CAD build for the part. Positions are in the model's coordinates, mm. Face numbers are marked on the shaded views. Give positions to 0.01 mm unless a question says otherwise; leave off trailing zeros. Answer as CSV lines item,"result".
from build123d import *

# Parameters (mm, degrees)
SKETCH_R        = 22.6
SKETCH_R_2      = 14
SKETCH_R_3      = 2.5
PAD_DEPTH       = 13
SKETCH001_R     = 27.5
SKETCH001_R_2   = 22.5
PAD001_DEPTH    = 2
CHAMFER_SIZE    = 0.5
CHAMFER001_SIZE = 1
CHAMFER002_SIZE = 0.5
CHAMFER003_SIZE = 0.5


with BuildPart() as part:
    # Sketch → Pad (new body)
    with BuildSketch(Plane.XY):
        Circle(SKETCH_R)
        Circle(SKETCH_R_2, mode=Mode.SUBTRACT)
        with Locations((0, 18)):
            Circle(SKETCH_R_3, mode=Mode.SUBTRACT)
        with Locations((-15.588457, -9)):
            Circle(SKETCH_R_3, mode=Mode.SUBTRACT)
        with Locations((15.588457, -9)):
            Circle(SKETCH_R_3, mode=Mode.SUBTRACT)
        with Locations((0, -18)):
            Circle(SKETCH_R_3, mode=Mode.SUBTRACT)
        with Locations((-15.588457, 9)):
            Circle(SKETCH_R_3, mode=Mode.SUBTRACT)
        with Locations((15.588457, 9)):
            Circle(SKETCH_R_3, mode=Mode.SUBTRACT)
        with Locations((-9, 15.588457)):
            Circle(SKETCH_R_3, mode=Mode.SUBTRACT)
        with Locations((9, -15.588457)):
            Circle(SKETCH_R_3, mode=Mode.SUBTRACT)
        with Locations((9, 15.588457)):
            Circle(SKETCH_R_3, mode=Mode.SUBTRACT)
        with Locations((-9, -15.588457)):
            Circle(SKETCH_R_3, mode=Mode.SUBTRACT)
        with Locations((18, 0)):
            Circle(SKETCH_R_3, mode=Mode.SUBTRACT)
        with Locations((-18, 0)):
            Circle(SKETCH_R_3, mode=Mode.SUBTRACT)
    extrude(amount=PAD_DEPTH)

    # Sketch001 (on Face15 of Pad) → Pad001 (join)
    with BuildSketch(Plane(origin=(0, 0, 0), x_dir=(1, 0, 0), z_dir=(0, 0, -1))):
        Circle(SKETCH001_R)
        Circle(SKETCH001_R_2, mode=Mode.SUBTRACT)
    extrude(amount=-PAD001_DEPTH)

    # Chamfer
    chamfer_edges = [part.edges().sort_by_distance(p)[0] for p in [
        (-27.5, 0, 2),
    ]]
    chamfer(chamfer_edges, length=CHAMFER_SIZE)

    # Chamfer001
    chamfer001_edges = [part.edges().sort_by_distance(p)[0] for p in [
        (-22.6, 0, 13),
    ]]
    chamfer(chamfer001_edges, length=CHAMFER001_SIZE)

    # Chamfer002
    chamfer002_edges = [part.edges().sort_by_distance(p)[0] for p in [
        (13.088457, -9, 13),
        (-11.5, 15.588457, 13),
        (-18.088457, 9, 13),
        (-11.5, -15.588457, 13),
        (6.5, 15.588457, 13),
        (-18.088457, -9, 13),
        (-2.5, 18, 13),
        (-20.5, 0, 13),
        (6.5, -15.588457, 13),
        (15.5, 0, 13),
        (-2.5, -18, 13),
        (13.088457, 9, 13),
    ]]
    chamfer(chamfer002_edges, length=CHAMFER002_SIZE)

    # Chamfer003
    chamfer003_edges = [part.edges().sort_by_distance(p)[0] for p in [
        (-14, 0, 13),
    ]]
    chamfer(chamfer003_edges, length=CHAMFER003_SIZE)


solid = part.part
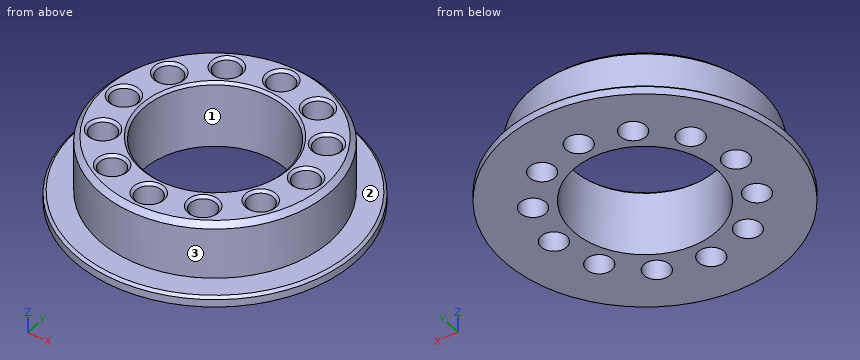
1) Flat gauge pins, fed straight in: pin 1 (25 mm diameter, centred on x = 0, y = 0, fed in from -Z); pin 2 (5 mm diameter, centred on x = 8.5, z = 9, fed in from +Y); pin 3 (2 mm diameter, centred on y = -20.5, z = 6.5, fed in from -X). Where does each tip first touch, or does it go through?
Answer below:
pin 1,"passes through"
pin 2,"stops at y = 21.79"
pin 3,"stops at x = -11.42"
2) Drill centre lines: line 1 (Y direction, x = 1, z = 10.75); line 2 (X direction, y = -16.5, z = 5.75). Where is each one in solid material? Low to high. Write a range as from..to.
Answer below:
line 1,"y = -22.58..-20.29, -15.71..-13.96, 13.96..15.71, 20.29..22.58"
line 2,"x = -15.44..-11.33, -6.67..-2, 2..6.67, 11.33..15.44"
3) Band-saw the part on A-A on x = 0. Give the number of separate pieces and of enclosed holes in the cut face, and give its area (3 significant figures).
Answer below:
separate pieces,"4"
enclosed holes,"0"
area,"111 mm^2"
4) Mould opens along Y. For the marked faces 1, 2 and 3 say: +Y half, -Y half, draft (parallel to the pull), parting line (faces both ways), or undercut.
Answer below:
face 1,"undercut"
face 2,"draft"
face 3,"parting line"
